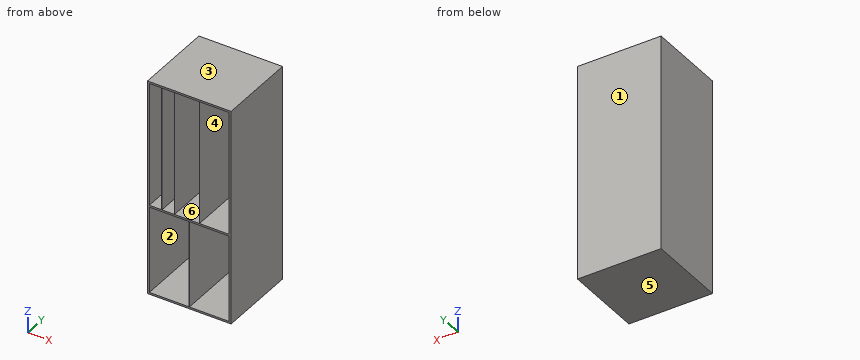
from build123d import *

# Parameters (mm, degrees)
F0_W     = 1.905
F0_H     = 889
F0_H_2   = 1270
F0_W_2   = 127
F0_H_3   = 19.05
F1_DEPTH = 812.8
F2_W     = 856.615
F2_H     = 2216.15
F3_DEPTH = 3.175


with BuildPart() as f1:
    # F0 (on Front) → F1 (new body)
    with BuildSketch(Plane.XZ):
        Polygon((-409.2575, 1079.5), (-409.2575, 1098.55), (-428.3075, 1098.55), (-428.3075, -1117.6), (-409.2575, -1117.6), (-409.2575, -1098.55), (-409.2575, -209.55), (-409.2575, -190.5), align=None)
        Polygon((-409.2575, -1098.55), (-409.2575, -1117.6), (409.2575, -1117.6), (409.2575, -1098.55), (0.9525, -1098.55), (-0.9525, -1098.55), align=None)
        Polygon((428.3075, 1098.55), (409.2575, 1098.55), (409.2575, 1079.5), (409.2575, 463.55), (409.2575, 419.1), (409.2575, -190.5), (409.2575, -209.55), (409.2575, -342.9), (409.2575, -1098.55), (409.2575, -1117.6), (428.3075, -1117.6), align=None)
        Polygon((-282.2575, -190.5), (-409.2575, -190.5), (-409.2575, -209.55), (-0.9525, -209.55), (0.9525, -209.55), (409.2575, -209.55), (409.2575, -190.5), (104.4575, -190.5), (102.5525, -190.5), (-151.4475, -190.5), (-153.3525, -190.5), (-280.3525, -190.5), align=None)
        with Locations((0, -654.05)):
            Rectangle(F0_W, F0_H)
        with Locations((-281.305, 444.5)):
            Rectangle(F0_W, F0_H_2)
        with Locations((-152.4, 444.5)):
            Rectangle(F0_W, F0_H_2)
        with Locations((103.505, 444.5)):
            Rectangle(F0_W, F0_H_2)
        Polygon((102.5525, 1098.55), (-153.3525, 1098.55), (-153.3525, 1079.5), (-151.4475, 1079.5), (102.5525, 1079.5), align=None)
        Polygon((409.2575, 1098.55), (102.5525, 1098.55), (102.5525, 1079.5), (104.4575, 1079.5), (409.2575, 1079.5), align=None)
        Polygon((-153.3525, 1098.55), (-282.2575, 1098.55), (-282.2575, 1079.5), (-280.3525, 1079.5), (-153.3525, 1079.5), align=None)
        with Locations((-345.7575, 1089.025)):
            Rectangle(F0_W_2, F0_H_3)
    extrude(amount=F1_DEPTH)

    # F2 (on face) → F3 (join)
    with BuildSketch(Plane(origin=(0, 0, 0), x_dir=(-1, 0, 0), z_dir=(0, 1, 0))):
        with Locations((0, -9.525)):
            Rectangle(F2_W, F2_H)
    extrude(amount=F3_DEPTH)


solid = f1.part
Geometry check sheet. Reference: the model listing, model coordinates, mm. Face numbers are marked on the shaded views. A direction names the side the tool comes from. Give positions to 0.01 mm unless a question says otherwise; leave off trailing zeros. Loops run counter-clockwise (first coordinate to the right, second up) from the corner with the lowest first, then second, coordinate; pieces in that order, holes last. Notation, with made-up numbers: M -32.5,61 L -19.5,61 A21 cw -19.5,93 Z; hole C 31.25,38.5 d5. An arc over 180 degrees is marked long. Answer as a JSON object with one key per item and string values. Group by question number.
Item 1: Access from +Z, -Z, +X, -X, +Y, -Y to the whole of each face (thin tool, end or side, straight path). Record for the marked faces 5 and 6.
Item 2: Sectioned sample at A-A on y = -540. Record the boundary of the cut face in (x, z).
Item 3: Material ranges on L1, parallel to Z at x = 335, y = -406.5; L2, parallel to X at y = -739.5, z = 403.5, recorded low to high.
Item 4: Sectioned sample at C-C on x = 310.5. Record the boundary of the cut face in (y, z) (3 decimals), plus the area to 3 significant figures.
Item 5: Gauge pin test, flat end, axial feed: pin 1 (1 mm diameter, centred on x = 322, z = -871, fed in from -Y). Record the tip position at first contact, or that the pin passes through.
Item 6: Mould release check, pull along Z, two halves, no side actions. Record for the marked faces 1, 2, 3 and 4: pulls with the +Z half, pulls with the -Z half, needs draft (parallel to the pull), parting line crosses it, or undercut.
Item 7: Sectioned sample at D-D on z = 870.5. Record the boundary of the cut face in (x, y) (1 decimal).
Item 8: Sectioned sample at B-B on z = -304.5. Record the boundary of the cut face in (x, y) (1 decimal).
Findings below:
{
 "1": {"face 5": "-Z, +X, -X, +Y, -Y", "face 6": "-Y"},
 "2": {"outline": "M -428.31,-1117.6 L 428.31,-1117.6 L 428.31,1098.55 L -428.31,1098.55 Z; hole M -409.26,-1098.55 L -0.95,-1098.55 L -0.95,-209.55 L -409.26,-209.55 Z; hole M -409.26,-190.5 L -282.26,-190.5 L -282.26,1079.5 L -409.26,1079.5 Z; hole M -280.35,-190.5 L -153.35,-190.5 L -153.35,1079.5 L -280.35,1079.5 Z; hole M -151.45,-190.5 L 102.55,-190.5 L 102.55,1079.5 L -151.45,1079.5 Z; hole M 0.95,-1098.55 L 409.26,-1098.55 L 409.26,-209.55 L 0.95,-209.55 Z; hole M 104.46,-190.5 L 409.26,-190.5 L 409.26,1079.5 L 104.46,1079.5 Z"},
 "3": {"L1": "-1117.6 to -1098.55, -209.55 to -190.5, 1079.5 to 1098.55", "L2": "-428.31 to -409.26, -282.26 to -280.35, -153.35 to -151.45, 102.55 to 104.46, 409.26 to 428.31"},
 "4": {"outline": "M -812.8,-1117.6 L 3.175,-1117.6 L 3.175,1098.55 L -812.8,1098.55 L -812.8,1079.5 L 0,1079.5 L 0,-190.5 L -812.8,-190.5 L -812.8,-209.55 L 0,-209.55 L 0,-1098.55 L -812.8,-1098.55 Z", "area": "53,500 mm2"},
 "5": {"pin 1": "y = 0"},
 "6": {"face 1": "needs draft", "face 2": "undercut", "face 3": "pulls with the +Z half", "face 4": "undercut"},
 "7": {"outline": "M -428.3,-812.8 L -409.3,-812.8 L -409.3,0 L -282.3,0 L -282.3,-812.8 L -280.4,-812.8 L -280.4,0 L -153.4,0 L -153.4,-812.8 L -151.4,-812.8 L -151.4,0 L 102.6,0 L 102.6,-812.8 L 104.5,-812.8 L 104.5,0 L 409.3,0 L 409.3,-812.8 L 428.3,-812.8 L 428.3,3.2 L -428.3,3.2 Z"},
 "8": {"outline": "M -428.3,-812.8 L -409.3,-812.8 L -409.3,0 L -1,0 L -1,-812.8 L 1,-812.8 L 1,0 L 409.3,0 L 409.3,-812.8 L 428.3,-812.8 L 428.3,3.2 L -428.3,3.2 Z"}
}
